Print and shaded views of the part. All mm, measured from the part's lowest x, y and z. A direction names the side the tool comes from. Round coordinates to 2 decimals unless told otherwise and drop trailing zeros. Write each loop counter-clockwise with the first axis right and the second up, starting at its lowest first coordinate (ties: lowest second). Pieces come first, ordered by that corner, then holes. Notation, with made-up numbers: (-40, 4.25) - (-6, 4.25) arc R21 cw to (-6, 10.25) - close; hole circle Ø10 at (4.25, -11). An arc over 180 degrees is marked (long way). Put each result on its own line as item: value. Start each with the question number.
Item 1: Cut at B-B (y = 40). Give the cut face in (x, z).
Item 2: Cut at C-C (z = 130). Give the cut face in (x, y).
Item 3: Pin check, flat tips, straight feed: pin 1 Ø6 at (x, y) = (74.5, 38.5) entering from +Z; pin 2 Ø5 at (x, y) = (51.5, 40.5) entering from -Z. Stop position of each tip, or through.
Item 4: 3-axis set-ups, long thin cutter, end or side, ignore diameter. For the marked faces 4 and 5: which of +Z, -Z, +X, -X, +Y, -Y reach the whole face in a straight line?
Item 5: Mould opens along Z. For the marked faces 1, 2 and 3 say: released by +Z, released by -Z, zero draft, split by the parting line, or undercut.
Item 6: Cut at A-A (x = 60). Give the cut face in (y, z).
Item 7: Cut at D-D (z = 14). Give the cut face in (x, y).
Item 8: Drill centre lines: line 1 (Y direction, x = 60, z = 11); line 2 (X direction, y = 48, z = 100); line 3 (Z direction, x = 61.5, y = 71). Where is each one in solid material? Low to high. Write a range as from..to.
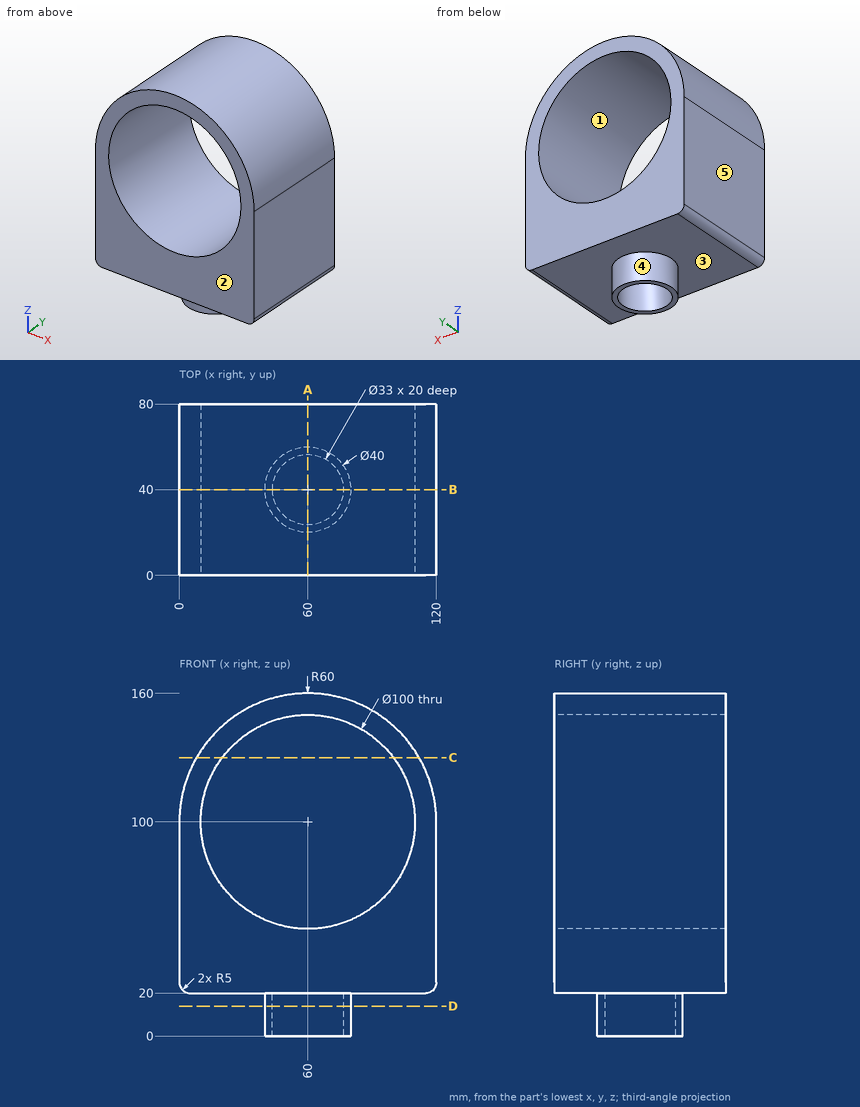
Output values:
1. outline: (0, 25) arc R5 ccw to (5, 20) - (40, 20) - (40, 0) - (43.5, 0) - (43.5, 20) - (76.5, 20) - (76.5, 0) - (80, 0) - (80, 20) - (115, 20) arc R5 ccw to (120, 25) - (120, 100) arc R60 ccw to (0, 100) - close; hole circle Ø100 at (60, 100)
2. outline: (8.04, 0) - (20, 0) - (20, 80) - (8.04, 80) - close; (100, 0) - (111.96, 0) - (111.96, 80) - (100, 80) - close
3. pin 1: z = 158.89
3. pin 2: z = 20
4. face 4: -Z
4. face 5: +Z, -Z, -X, +Y, -Y
5. face 1: undercut
5. face 2: zero draft
5. face 3: released by -Z
6. outline: (0, 20) - (20, 20) - (20, 0) - (23.5, 0) - (23.5, 20) - (56.5, 20) - (56.5, 0) - (60, 0) - (60, 20) - (80, 20) - (80, 50) - (0, 50) - close; (0, 150) - (80, 150) - (80, 160) - (0, 160) - close
7. outline: circle Ø40 at (60, 40); hole circle Ø33 at (60, 40)
8. line 1: 20..23.5, 56.5..60
8. line 2: 0..10, 110..120
8. line 3: 20..50.02, 149.98..159.98
